Study the drawing (mm; zero at the part's minimum x, y, z) and answer. Coordinates: 2 decimals unless noted, no trailing zeros. Loops run counter-clockwise (first coordinate to the right, second up) from the corner with the lowest first, then second, coordinate; pieces in that order, holes last. Notation, with made-up numbers: (84.5, 19) -> (126.5, 19) arc R19 ccw to (126.5, 45) -> close; hole circle Ø11 at (64, 3.25). An arc over 180 degrees is marked (long way). Answer as a JSON object with one key per item and string values. Group by question number.
Q1. Determine the mould class of the marked faces 1, 2 and 3 for opening direction Z: released by +Z, released by -Z, zero draft, split by the parting line, or undercut.
Q2. The part is cut by section A-A on z = 47.5. Write down the section's boundary in (x, y).
Q3. The part is cut by section C-C on y = 17.25. Write down the section's boundary in (x, z).
Q4. The part is cut by section D-D on x = 20. Write down the section's boundary in (y, z).
Q5. Straight lines are drawn through the part: line 1 along X through (y, z) = (6.5, 47.5); line 2 along Z through (x, y) = (41, 14.75); line 3 along X through (y, z) = (13.25, 45.5). For each, find the intervals that lie inside material, in ascending order. Write a range as [from, to].
Q6. The part is cut by section B-B on x = 40. Write down the section's boundary in (y, z).
Q7. Each of these flat-tipped pins is pushed along its axis until it touches: P1, Ø8, axis at x = 42, y = 13, coming from the -Z side; P2, Ø1.5, axis at y = 10.5, z = 30.5, coming from the +X side; P3, Ø10, axis at x = 56.5, y = 17.5, coming from the -Z side. Where does it stop, or does it pass through?
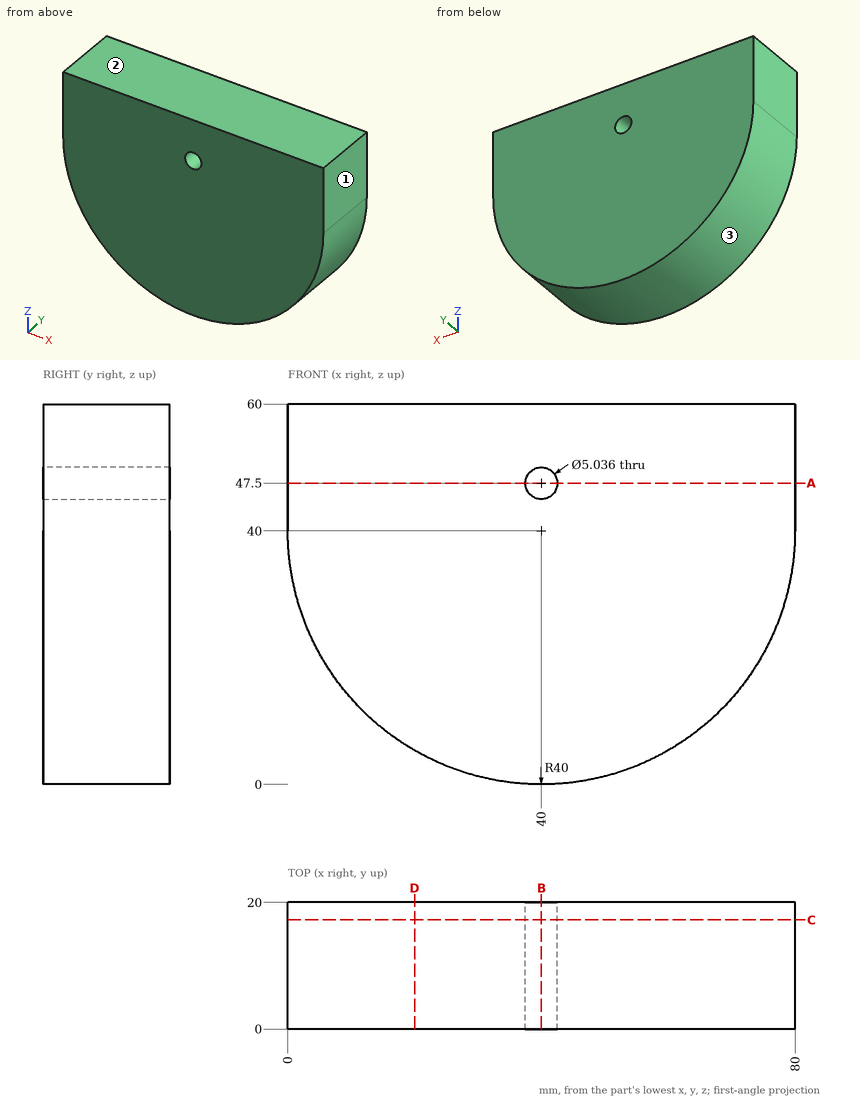
Final values:
{
 "1": {"face 1": "zero draft", "face 2": "released by +Z", "face 3": "released by -Z"},
 "2": {"outline": "(0, 0) -> (37.48, 0) -> (37.48, 20) -> (0, 20) -> close; (42.52, 0) -> (80, 0) -> (80, 20) -> (42.52, 20) -> close"},
 "3": {"outline": "(0, 40) arc R40 ccw to (80, 40) -> (80, 60) -> (0, 60) -> close; hole circle Ø5.04 at (40, 47.5)"},
 "4": {"outline": "(0, 5.36) -> (20, 5.36) -> (20, 60) -> (0, 60) -> close"},
 "5": {"line 1": "x = [0, 37.48], [42.52, 80]", "line 2": "z = [0.01, 45.19], [49.81, 60]", "line 3": "x = [0, 38.47], [41.53, 80]"},
 "6": {"outline": "(0, 0) -> (20, 0) -> (20, 44.98) -> (0, 44.98) -> close; (0, 50.02) -> (20, 50.02) -> (20, 60) -> (0, 60) -> close"},
 "7": {"P1": "stops at z = 0", "P2": "stops at x = 79.03", "P3": "stops at z = 1.69"}
}
